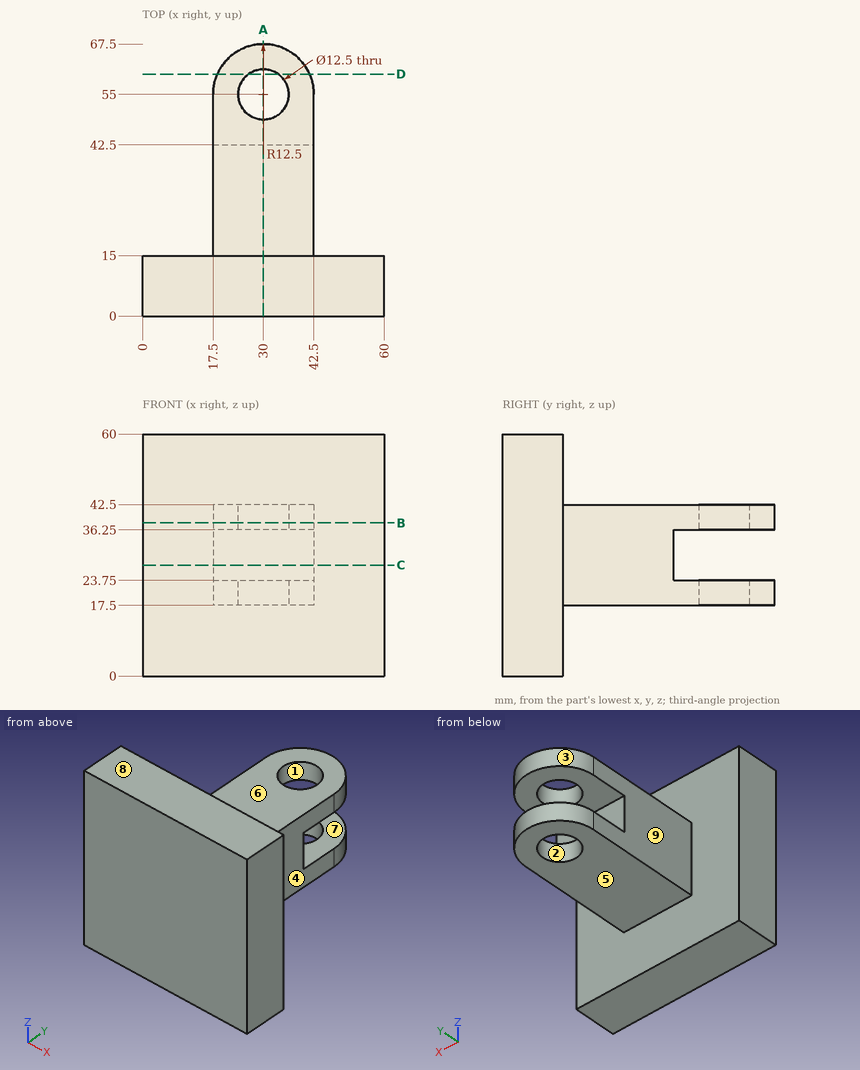
Print and shaded views of the part. All mm, measured from the part's lowest x, y and z. A direction names the side the tool comes from. Give positions to 0.01 mm unless a question says otherwise; leave off trailing zeros. Loops run counter-clockwise (first coordinate to the right, second up) from the corner with the lowest first, then second, coordinate; pieces in that order, holes last. Notation, with made-up numbers: M 79.25,-17.75 L 89.25,-17.75 A14 ccw 89.25,1.25 Z; hole C -8,87.5 d2. An arc over 180 degrees is marked long. Write each question's results on one line, items separated by ' | '.
Q1. Band-saw the part on B-B on z = 38. Write the cut outline in (x, y).
Geometry check:
outline: M 0,0 L 60,0 L 60,15 L 42.5,15 L 42.5,55 A12.5 ccw 17.5,55 L 17.5,15 L 0,15 Z; hole C 30,55 d12.5
Q2. Band-saw the part on A-A on x = 30. Write the cut outline in (y, z), and give its area (3 significant figures).
Geometry check:
outline: M 0,0 L 15,0 L 15,17.5 L 48.75,17.5 L 48.75,23.75 L 42.5,23.75 L 42.5,36.25 L 48.75,36.25 L 48.75,42.5 L 15,42.5 L 15,60 L 0,60 Z; M 61.25,17.5 L 67.5,17.5 L 67.5,23.75 L 61.25,23.75 Z; M 61.25,36.25 L 67.5,36.25 L 67.5,42.5 L 61.25,42.5 Z | area: 1,740 mm²
Q3. Mould opens along Y. For the marked faces 1, 2, 3 and 4 say: pulls with the +Y half, pulls with the -Y half, needs draft (parallel to the pull), parting line crosses it, or undercut.
Geometry check:
face 1: undercut | face 2: undercut | face 3: pulls with the +Y half | face 4: needs draft
Q4. Band-saw the part on C-C on z = 27.5. Write the cut outline in (x, y).
Geometry check:
outline: M 0,0 L 60,0 L 60,15 L 42.5,15 L 42.5,42.5 L 17.5,42.5 L 17.5,15 L 0,15 Z
Q5. Probe probe 1 along Y at (x, z) = (30, 38); probe 2 along X at (y, z) = (55, 20.5). List the from-to ranges inside material, lowest first.
Geometry check:
probe 1: y = 0 to 48.75, 61.25 to 67.5 | probe 2: x = 17.5 to 23.75, 36.25 to 42.5
Q6. Band-saw the part on D-D on y = 60. Write the cut outline in (x, z), and give its area (3 significant figures).
Geometry check:
outline: M 18.54,17.5 L 26.25,17.5 L 26.25,23.75 L 18.54,23.75 Z; M 18.54,36.25 L 26.25,36.25 L 26.25,42.5 L 18.54,42.5 Z; M 33.75,17.5 L 41.46,17.5 L 41.46,23.75 L 33.75,23.75 Z; M 33.75,36.25 L 41.46,36.25 L 41.46,42.5 L 33.75,42.5 Z | area: 193 mm²
Q7. Which spindle directions (+Z, -Z, +X, -X, +Y, -Y) get a long thin tool onto all of the face, cutting with end or side? Do the marked faces 5, 6, 7, 8 and 9. Say none if no direction does.
Geometry check:
face 5: -Z, +X, -X, +Y | face 6: +Z, +X, -X, +Y | face 7: +X, -X, +Y | face 8: +Z, +X, -X, +Y, -Y | face 9: +Z, -Z, -X, +Y
Q8. Flat gauge pins, fed straight in: P1, Ø3, axis at x = 20, y = 50.5, coming from the +Z side; P2, Ø8, axis at x = 13, z = 33.5, coming from the +Y side; P3, Ø20, axis at x = 31, y = 56, coming from the -Z side. Where does each tip first touch, or does it go through?
Geometry check:
P1: stops at z = 42.5 | P2: stops at y = 15 | P3: stops at z = 17.5
